Autodesk Inventor part; units mm, degrees
ref_plane "YZ Plane" through (0, 0, 0) normal (1, 0, 0) x (0, 1, 0)
ref_plane "XZ Plane" through (0, 0, 0) normal (0, 1, 0) x (-1, 0, 0)
ref_plane "XY Plane" through (0, 0, 0) normal (0, 0, 1) x (1, 0, 0)
sketch "Sketch1" plane through (0, 0, 0) normal (0, 0, 1) x (1, 0, 0)
  line L0 (-63.5, 63.5) -> (63.5, 63.5)
  line L1 (63.5, 63.5) -> (63.5, -63.5)
  line L2 (63.5, -63.5) -> (-63.5, -63.5)
  line L3 (-63.5, -63.5) -> (-63.5, 63.5)
  circle A0 centre (-57.15, 57.15) radius 1.524
  circle A1 centre (57.15, 57.15) radius 1.524
  line L4 (63.5, 0) -> (-63.5, 0)
  circle A2 centre (-57.15, -57.15) radius 1.524
  circle A3 centre (57.15, -57.15) radius 1.524
  point P0 (0, 0)
  point P1 (0, 63.5)
  dimension "d0" = 127
  dimension "d1" = 127
  dimension "d2" = 127
  dimension "d3" = 3.048
  dimension "d4" = 3.048
  dimension "d5" = 6.35
  dimension "d6" = 6.35
  dimension "d7" = 6.35
  dimension "d8" = 6.35
extrude "Extrusion1" add sketch "Sketch1" along normal blind 3.175
sketch "Sketch2" plane through (0, 0, 3.175) normal (0, 0, 1) x (1, 0, 0)
  circle A0 centre (0, 0) radius 3.81
  circle A1 centre (-15.494, 15.494) radius 1.524
  circle A2 centre (15.494, 15.494) radius 1.524
  circle A3 centre (-15.494, -15.494) radius 1.524
  circle A4 centre (15.494, -15.494) radius 1.524
  line L0 (-15.494, 15.494) -> (15.494, 15.494)
  line L1 (-15.494, -15.494) -> (-15.494, 15.494)
  point P0 (0, 15.494)
  point P1 (-15.494, 0)
  dimension "d11" = 7.62
  dimension "d12" = 3.048
  dimension "d13" = 3.048
  dimension "d14" = 3.048
  dimension "d15" = 3.048
  dimension "d16" = 30.988
  dimension "d21" = 30.988
  dimension "d22" = 30.988
extrude "Extrusion2" cut sketch "Sketch2" against normal blind 25.4
fillet "Fillet1" radius 3.175 4 edges at (0, 63.5, 0) (-63.5, 0, 0) (0, -63.5, 0) (63.5, 0, 0)
sketch "Sketch4" plane through (0, 0, 0) normal (0, 0, -1) x (-1, 0, 0)
  circle A0 centre (0, 0) radius 3.81
  line L0 (0, 0) -> (50.8, 0)
  line L1 (60.325, 60.325) -> (60.325, -60.325)
  line L2 (-60.325, 60.325) -> (60.325, 60.325)
  line L3 (0, 60.325) -> (60.325, 60.325)
  line L4 (63.5, 63.5) -> (63.5, -63.5)
  line L5 (60.325, 60.325) -> (60.325, 47.625)
  line L6 (25.4, 0) -> (25.4, 47.625)
  circle A1 centre (25.4, 47.625) radius 3.75
  circle A2 centre (50.8, 0) radius 3.75
  circle A3 centre (25.4, -47.625) radius 3.75
  line L7 (25.4, 47.625) -> (50.8, 0)
  line L8 (50.8, 0) -> (25.4, -47.625)
  line L9 (27.0544, 48.5074) -> (52.925, 0)
  line L10 (52.925, 0) -> (27.0544, -48.5074)
  line L11 (23.7456, 46.7426) -> (48.675, 0)
  line L12 (48.675, 0) -> (23.7456, -46.7426)
  circle A4 centre (15.494, 15.494) radius 1.524
  line L13 (15.494, 0) -> (7.747, -13.4182)
  line L14 (7.747, -13.4182) -> (-7.747, -13.4182)
  line L15 (-7.747, -13.4182) -> (-15.494, 0)
  line L16 (-15.494, 0) -> (-7.747, 13.4182)
  line L17 (-7.747, 13.4182) -> (7.747, 13.4182)
  line L18 (7.747, 13.4182) -> (15.494, 0)
  line L19 (0, 60.325) -> (0, 13.4182)
  line L20 (0, 0) -> (-50.8, 0)
  line L21 (-25.4, 0) -> (-25.4, 47.625)
  circle A5 centre (-25.4, 47.625) radius 3.75
  circle A6 centre (-50.8, 0) radius 3.75
  circle A7 centre (-25.4, -47.625) radius 3.75
  line L22 (-25.4, 47.625) -> (-50.8, 0)
  line L23 (-50.8, 0) -> (-25.4, -47.625)
  line L24 (-27.0544, 48.5074) -> (-52.925, 0)
  line L25 (-52.925, 0) -> (-27.0544, -48.5074)
  line L26 (-23.7456, 46.7426) -> (-48.675, 0)
  line L27 (-48.675, 0) -> (-23.7456, -46.7426)
  circle A8 centre (-15.494, 15.494) radius 1.524
  point P0 (-25.4, 43.875)
  point P1 (-28.5827, 45.6418)
  point P2 (-50.9261, 3.7479)
  point P3 (-50.9261, -3.7479)
  point P4 (-28.5827, -45.6418)
  point P5 (-25.2739, -43.8771)
  point P6 (-47.6173, -1.9832)
  point P7 (-47.6173, 1.9832)
  point P8 (-25.4, 43.6406)
  point P9 (50.9261, 3.7479)
  point P10 (28.5827, 45.6418)
  point P11 (25.4, 43.875)
  point P12 (25.4, 43.6406)
  point P13 (47.6173, 1.9832)
  point P14 (47.6173, -1.9832)
  point P15 (25.2739, -43.8771)
  point P16 (28.5827, -45.6418)
  point P17 (50.9261, -3.7479)
  dimension "d24" = 50.8
  dimension "d25" = 12.7
  dimension "d26" = 7.5
  dimension "d27" = 7.5
  dimension "d28" = 1.875
  dimension "d29" = 1.875
extrude "Extrusion3" cut sketch "Sketch4" against normal blind 1 contours L0 L13 L14 L15 L20 A0 | A0 L20 L16 L17 L18 L0 | A2 L11 L0 | L0 L12 A2 | L6 A1 L7 A2 L11 | A6 L27 L20 | L20 L26 A6 | L26 A6 L22 A5 L21 | L11 A2 L7 L0 | L0 L8 A2 L12 | A2 L8 A3 L12 | A1 L7 L6 | L6 L7 A1 | L27 A6 L23 L20 | L20 L22 A6 L26 | L27 A7 L23 A6 | A5 L22 L21 | L21 L22 A5 | L7 A2 L9 L10 L8 | L7 A1 L9 A2 | A2 L10 A3 L8 | A3 | L23 A6 L25 L24 L22 | A6 L24 A5 L22 | L23 A7 L25 A6 | A7 | A2 L10 L9 | L24 L25 A6
sketch "Sketch5" plane through (0, 0, 0) normal (0, 0, -1) x (-1, 0, 0)
  line L0 (-7.747, 13.4182) -> (7.747, 13.4182)
  line L1 (7.747, 13.4182) -> (-7.747, 13.4182)
  point P0 (0, 0)
properties part number "base 2"
The listing builds one solid part. Answer for the finished solid, in the listing's coordinates (mm). A direction names the side the tool comes from. Coordinates: 2 decimals unless noted, no trailing zeros. Answer as CSV lines item,"result".
1. Straight lines are drawn through the part: line 1 (Y direction, x = 57, z = 2.8); line 2 (X direction, y = 2, z = 0.8); line 3 (Y direction, x = 57.15, z = 1.5). For each, find the intervals that lie inside material, in ascending order. Write a range as [from, to].
Computed values:
line 1,"y = [-63.48, -58.67], [-55.63, 55.63], [58.67, 63.48]"
line 2,"x = [-62.43, -53.97], [-47.61, -14.34], [14.34, 47.61], [53.97, 62.43]"
line 3,"y = [-63.02, -58.67], [-55.63, 55.63], [58.67, 63.02]"
2. A tool of negligible diameter and unlimited length cuts with its end or side. For faces 1 (the cylindrical face through (23.758, -50.996, 0.493)), 2 (the cylindrical face through (-56.447, -55.798, 1.565)), from which of +Z, -Z, +X, -X, +Y, -Y can it reach the whole face along a straight path? Write none if from no direction.
Computed values:
face 1,"-Z"
face 2,"+Z, -Z"
3. Given P1, Ø1, axis at x = 6, z = 0.5, coming from the -Y side; P2, Ø8.5, axis at x = 25.4, y = 47.625, coming from the -Z side; P3, Ø7, axis at x = -25.4, y = -47.625, coming from the -Z side, each flat-ended and moving along its own axis, determine where each tip first touches the part or whether it passes through.
Computed values:
P1,"stops at y = -62.64"
P2,"stops at z = 0"
P3,"stops at z = 1"
4. Find section B-B (x = 57.15). Give the number of separate pieces and of enclosed holes in the cut face, plus the area to 3 significant figures.
Computed values:
separate pieces,"3"
enclosed holes,"0"
area,"380 mm²"
5. Determine the mould class of faces 3 (the flat face through (-1, 14, 0)), 4 (the cylindrical face through (55.941, 58.077, 1.565)) for opening direction Y: +Y half, -Y half, draft (parallel to the pull), parting line (faces both ways), or undercut.
Computed values:
face 3,"draft"
face 4,"undercut"
